```python
from build123d import *

# Parameters (mm, degrees)
SKETCH1_R               = 10.2
BOSS_EXTRUDE1_DEPTH     = 2
CUT_EXTRUDE4_DEPTH      = 168.619360457
CUT_EXTRUDE4_DEPTH_BACK = 168.619360457
SKETCH5_W               = 20
SKETCH5_H               = 2


with BuildPart() as part:
    # Sketch1 → Boss-Extrude1 (new body)
    with BuildSketch(Plane.XY):
        Polygon((-156.5, -56), (-145.5, -56), (-145.5, -60), (-125.5, -60), (-125.5, -56), (-100.5, -56), (-100.5, -60), (-80.5, -60), (-80.5, -56), (-55.5, -56), (-55.5, -60), (-35.5, -60), (-35.5, -56), (35.5, -56), (35.5, -60), (55.5, -60), (55.5, -56), (80.5, -56), (80.5, -60), (100.5, -60), (100.5, -56), (125.5, -56), (125.5, -60), (145.5, -60), (145.5, -56), (156.5, -56), (156.5, -24), (154.5, -24), (154.5, -4), (156.5, -4), (156.5, 16), (154.5, 16), (154.5, 36), (156.5, 36), (156.5, 56), (145.5, 56), (145.5, 58), (125.5, 58), (125.5, 56), (100.5, 56), (100.5, 58), (80.5, 58), (80.5, 56), (55.5, 56), (55.5, 58), (35.5, 58), (35.5, 56), (-35.5, 56), (-35.5, 58), (-55.5, 58), (-55.5, 56), (-80.5, 56), (-80.5, 58), (-100.5, 58), (-100.5, 56), (-125.5, 56), (-125.5, 58), (-145.5, 58), (-145.5, 56), (-156.5, 56), (-156.5, 36), (-154.5, 36), (-154.5, 16), (-156.5, 16), (-156.5, -4), (-154.5, -4), (-154.5, -24), (-156.5, -24), align=None)
        with Locations((-66.5, -36)):
            Circle(SKETCH1_R, mode=Mode.SUBTRACT)
        with Locations((-26.5, -36)):
            Circle(SKETCH1_R, mode=Mode.SUBTRACT)
        with Locations(Location((26.5, -36, 0), (0, 0, 180))):
            Circle(SKETCH1_R, mode=Mode.SUBTRACT)
        with Locations(Location((66.5, -36, 0), (0, 0, 180))):
            Circle(SKETCH1_R, mode=Mode.SUBTRACT)
    extrude(amount=BOSS_EXTRUDE1_DEPTH)

    # Sketch5 → Cut-Extrude4 (cut, two sides: drawn at the far end of the back side and taken through both)
    with BuildSketch(Plane.XY.offset(2).offset(-CUT_EXTRUDE4_DEPTH_BACK)):
        with Locations((-135.5, 57)):
            Rectangle(SKETCH5_W, SKETCH5_H)
        with Locations((-90.5, 57)):
            Rectangle(SKETCH5_W, SKETCH5_H)
        with Locations((-45.5, 57)):
            Rectangle(SKETCH5_W, SKETCH5_H)
        with Locations((45.5, 57)):
            Rectangle(SKETCH5_W, SKETCH5_H)
        with Locations((90.5, 57)):
            Rectangle(SKETCH5_W, SKETCH5_H)
        with Locations((135.5, 57)):
            Rectangle(SKETCH5_W, SKETCH5_H)
    extrude(amount=CUT_EXTRUDE4_DEPTH + CUT_EXTRUDE4_DEPTH_BACK, mode=Mode.SUBTRACT)


solid = part.part
```
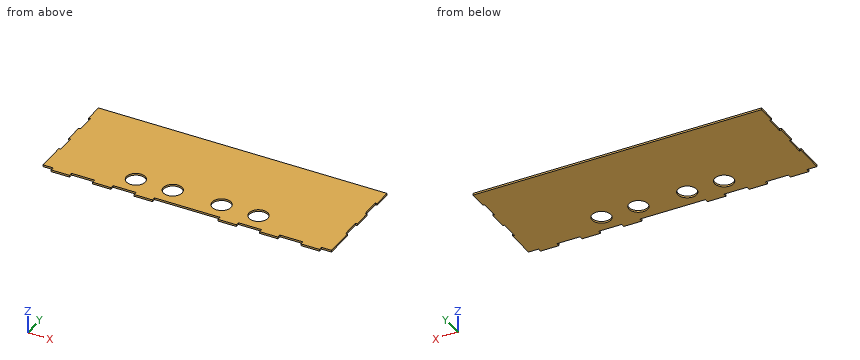
Read the model definition and answer for the solid it produces. Units are mm, in the model's axes. Coordinates: 2 decimals unless noted, no trailing zeros. Loops run counter-clockwise (first coordinate to the right, second up) from the corner with the lowest first, then second, coordinate; pieces in that order, holes last. Notation, with made-up numbers: (7.5, 7.25) -> (34.5, 7.25) arc R17 ccw to (34.5, 25.25) -> close; hole circle Ø8 at (24.5, 67). An arc over 180 degrees is marked (long way). Return JSON: item names as keys, results as strings.
Item 1: Find the intervals of material crossed by probe 1 along Y at (x, z) = (-66.5, 0.75); probe 2 along X at (y, z) = (-37, 0.55); probe 3 along X at (y, z) = (-29, 1.25), in increasing order.
Answers:
{"probe 1": "y = -56 to -46.2, -25.8 to 56", "probe 2": "x = -156.5 to -76.65, -56.35 to -36.65, -16.35 to 16.35, 36.65 to 56.35, 76.65 to 156.5", "probe 3": "x = -156.5 to -73.92, -59.08 to -33.92, -19.08 to 19.08, 33.92 to 59.08, 73.92 to 156.5"}
Item 2: Flat-ended cylindrical pins translate along their axes: P1, Ø1, axis at x = 156, z = 0.5, coming from the -Y side; P2, Ø1, axis at y = -57.5, z = 1.5, coming from the +X side; P3, Ø1, axis at y = -59, z = 1, coming from the -X side. Find the tip coordinate at first contact, or state that the pin passes through.
Answers:
{"P1": "stops at y = -56", "P2": "stops at x = 145.5", "P3": "stops at x = -145.5"}
Item 3: Find section A-A (y = -36). Determine the outline of the cut face in (x, z).
Answers:
{"outline": "(-156.5, 0) -> (-76.7, 0) -> (-76.7, 2) -> (-156.5, 2) -> close; (-56.3, 0) -> (-36.7, 0) -> (-36.7, 2) -> (-56.3, 2) -> close; (-16.3, 0) -> (16.3, 0) -> (16.3, 2) -> (-16.3, 2) -> close; (36.7, 0) -> (56.3, 0) -> (56.3, 2) -> (36.7, 2) -> close; (76.7, 0) -> (156.5, 0) -> (156.5, 2) -> (76.7, 2) -> close"}
Item 4: Find section C-C (z = 0.7). Count the separate pieces of the cut face and the enclosed holes in it, plus the area to 3 significant figures.
Answers:
{"separate pieces": "1", "enclosed holes": "4", "area": "34,100 mm2"}
Item 5: Find section B-B (x = 66.5). Determine the outline of the cut face in (y, z), plus the area to 3 significant figures.
Answers:
{"outline": "(-56, 0) -> (-46.2, 0) -> (-46.2, 2) -> (-56, 2) -> close; (-25.8, 0) -> (56, 0) -> (56, 2) -> (-25.8, 2) -> close", "area": "183 mm2"}
Item 6: Find section D-D (x = 5.5). Determine the outline of the cut face in (y, z).
Answers:
{"outline": "(-56, 0) -> (56, 0) -> (56, 2) -> (-56, 2) -> close"}
